from build123d import *

# Parameters (mm, degrees)
SKETCH1_R           = 6.049999999999999
SKETCH1_R_2         = 4.118749999999998
SKETCH1_R_3         = 4.118750000000009
SKETCH1_R_4         = 4.118750000000003
SKETCH1_R_5         = 4.11875000000001
BOSS_EXTRUDE1_DEPTH = 3
FILLET1_R           = 21.5
FILLET2_R           = 52
CUT_EXTRUDE1_DEPTH  = 189.18607812481773


with BuildPart() as part:
    # Sketch1 → Boss-Extrude1 (new, symmetric)
    with BuildSketch(Plane.XY):
        Polygon((0, 0), (0, 133), (42.999999999999986, 133), (133, 42.99999999999999), (133, 9.06e-15), align=None)
        with Locations((21.5, 21.499999999999993)):
            Circle(SKETCH1_R, mode=Mode.SUBTRACT)
        with Locations((21.5, 111.50000000000001)):
            Circle(SKETCH1_R_2, mode=Mode.SUBTRACT)
        with Locations((111.50000000000001, 21.5)):
            Circle(SKETCH1_R_3, mode=Mode.SUBTRACT)
        with Locations((21.5, 52.78839999999999)):
            Circle(SKETCH1_R_4, mode=Mode.SUBTRACT)
        with Locations((52.788399999999996, 21.499999999999986)):
            Circle(SKETCH1_R_5, mode=Mode.SUBTRACT)
    extrude(amount=BOSS_EXTRUDE1_DEPTH, both=True)

    # Fillet1
    fillet1_edges = [part.edges().sort_by_distance(p)[0] for p in [
        (0, 0, 0),
        (0, 133, 0),
        (133, 9.06e-15, 0),
    ]]
    fillet(fillet1_edges, radius=FILLET1_R)

    # Fillet2
    # the kernel refuses this fillet: 52 mm, written as the material it takes off along each edge
    with BuildSketch(Plane(origin=(133, 43, -56.84767436170304), x_dir=(-0.7071067811865476, 0.7071067811865476, 0), z_dir=(0, 0, 1))) as fillet2_piece_1:
        with BuildLine():
            CenterArc((21.539069744681207, 52.00000000000001), FILLET2_R, 225.07350833515432, 44.926491664845685)
            Line((-15.183278672480162, 15.183303696167892), (-18.855513514196304, 11.501634065784673))
            ThreePointArc((-18.855513514196304, 11.501634065784673), (-18.87975105768081, 11.52584053334073), (-3.6769552621700394, -3.6769552621700394))
            Line((-3.6769552621700394, -3.6769552621700394), (-4.9e-15, -5.200000000000005))
            Line((-4.9e-15, -5.200000000000005), (21.539069744681218, -5.199999999999996))
            Line((21.539069744681218, -5.199999999999996), (21.539069744681214, 4.7e-16))
        make_face()
    extrude(amount=113.69534872340608, mode=Mode.SUBTRACT)
    with BuildSketch(Plane(origin=(42.999999999999986, 133, 56.847674361702985), x_dir=(-0.9999999999996605, -8.240534738615283e-07, 0), z_dir=(0, 0, -1))) as fillet2_piece_2:
        with BuildLine():
            CenterArc((21.539173195539043, -51.9999571492017), FILLET2_R, 90.07355554994047, 44.926491664845685)
            Line((-15.230409726226513, -15.230434827591285), (-18.90736801840307, -11.55348259543025))
            Line((-18.90736801840307, -11.55348259543025), (-3.676958292176556, 3.6769522321610486))
            Line((-3.676958292176556, 3.6769522321610486), (-4.28507806408e-06, 5.199999999998223))
            ThreePointArc((-4.28507806408e-06, 5.199999999998223), (21.499995714914625, 5.200017717147912), (21.46574062621809, 5.1999957149201785))
            Line((21.46574062621809, 5.1999957149201785), (21.472416314338172, 0))
        make_face()
    extrude(amount=113.69534872340597, mode=Mode.SUBTRACT)

    # Sketch2 → Cut-Extrude1 (cut, through all)
    with BuildSketch(Plane.XY.offset(3)):
        with BuildLine():
            Line((117.76956733680983, 58.23043266319015), (58.23043266319017, 117.76956733680981))
            ThreePointArc((58.23043266319017, 117.76956733680981), (41.3784881824358, 129.03426172642116), (21.499999999999996, 133))
            ThreePointArc((21.499999999999996, 133), (6.2972042044892405, 126.70279579551078), (3.47e-15, 111.50000000000001))
            Line((3.47e-15, 111.50000000000001), (0, 21.5))
            ThreePointArc((0, 21.5), (6.297204204489223, 6.297204204489235), (21.49999999999999, 3.47e-15))
            Line((21.49999999999999, 3.47e-15), (111.50000000000001, 1.041e-14))
            ThreePointArc((111.50000000000001, 1.041e-14), (126.70279579551078, 6.297204204489239), (133, 21.500000000000007))
            ThreePointArc((133, 21.500000000000007), (129.03426172642114, 41.37848818243579), (117.76956733680983, 58.23043266319015))
        make_face()
        with BuildLine():
            Line((114.94114021206362, 55.40200553844396), (55.402005538443966, 114.94114021206363))
            ThreePointArc((55.402005538443966, 114.94114021206363), (39.84708125964561, 125.33902242576387), (21.49854269401705, 128.9999999393217))
            ThreePointArc((21.49854269401705, 128.9999999393217), (9.12511610449009, 123.87385342456624), (4.0000000000000036, 111.50000000000001))
            Line((4.0000000000000036, 111.50000000000001), (4, 21.500000000000004))
            ThreePointArc((4, 21.500000000000004), (9.125631329235414, 9.125631329235425), (21.499999999999996, 4.0000000000000036))
            Line((21.499999999999996, 4.0000000000000036), (111.50000000000001, 4.000000000000011))
            ThreePointArc((111.50000000000001, 4.000000000000011), (123.8738534245646, 9.125116104488455), (128.9999999393217, 21.49854269401244))
            ThreePointArc((128.9999999393217, 21.49854269401244), (125.33902242576474, 39.847081259643474), (114.94114021206362, 55.40200553844396))
        make_face(mode=Mode.SUBTRACT)
    extrude(amount=-CUT_EXTRUDE1_DEPTH, mode=Mode.SUBTRACT)


with BuildPart() as cut_extrude1_kept_piece:
    # of the separate pieces the step leaves, the one the design keeps (cut_extrude1_pieces_kept)
    add(part.part.solids().sort_by_distance((128.999999939, 21.498542694, -3))[0])


solid = cut_extrude1_kept_piece.part
Could you check a few things on this model? Use its own coordinates, in mm. Coordinates: 2 decimals unless noted, no trailing zeros. Loops run counter-clockwise (first coordinate to the right, second up) from the corner with the lowest first, then second, coordinate; pieces in that order, holes last. Notation, with made-up numbers: (9, 13.25) -> (65, 13.25) arc R27 cw to (65, 47.25) -> close; hole circle Ø1 at (46, -7.75). An arc over 180 degrees is marked (long way). Answer in a Markdown table with one row per item.
(1) If I drill on probe 1 along Y at (x, z) = (21.5, -0.45); probe 2 along Y at (x, z) = (88.5, -1.6); probe 3 along Y at (x, z) = (94, 1.2), over which ranges is the centre line in solid material (lowest first)?
Results found:
| item | result |
|---|---|
| probe 1 | y = 4 to 15.45, 27.55 to 48.67, 56.91 to 107.38, 115.62 to 129 |
| probe 2 | y = 4 to 81.84 |
| probe 3 | y = 4 to 76.34 |
(2) Imagine slicing it at A-A (z = 2). List the corners of the cut face in (x, y) for me.
Results found:
| item | result |
|---|---|
| outline | (4, 21.5) arc R17.5 ccw to (21.5, 4) -> (111.5, 4) arc R17.5 ccw to (129, 21.5) arc R48 ccw to (114.94, 55.4) -> (55.4, 114.94) arc R48 ccw to (21.5, 129) arc R17.5 ccw to (4, 111.5) -> close; hole circle Ø12.1 at (21.5, 21.5); hole circle Ø8.24 at (21.5, 52.79); hole circle Ø8.24 at (21.5, 111.5); hole circle Ø8.24 at (52.79, 21.5); hole circle Ø8.24 at (111.5, 21.5) |
(3) Thinking about a two-plate mould opening in X: for faces 1 (the face through (20.607, 48.768, -0.042)), 2 (the face through (53, 53, -3)), 3 (the face through (123.74, 8.99, 0.04)), which applies, released by +X, released by -X, zero draft, split by the parting line, or undercut?
Results found:
| item | result |
|---|---|
| face 1 | undercut |
| face 2 | zero draft |
| face 3 | released by +X |
(4) Imagine slicing it at C-C (y = 99). List the corners of the cut face in (x, z) for me.
Results found:
| item | result |
|---|---|
| outline | (4, -3) -> (71.34, -3) -> (71.34, 3) -> (4, 3) -> close |
(5) Imagine slicing it at B-B (x = 97.5). List the corners of the cut face in (y, z) for me.
Results found:
| item | result |
|---|---|
| outline | (4, -3) -> (72.84, -3) -> (72.84, 3) -> (4, 3) -> close |
